from build123d import *

# Parameters (mm, degrees)
F0_R     = 3
F0_R_2   = 1.5
F1_DEPTH = 2
F2_DEPTH = 7
F3_SIZE  = 1


with BuildPart() as f1:
    # F0 (on Top) → F1 (new body)
    with BuildSketch(Plane.XY):
        Circle(F0_R)
        Circle(F0_R_2, mode=Mode.SUBTRACT)
    extrude(amount=F1_DEPTH)

    # F0 (on Top) → F2 (join)
    with BuildSketch(Plane.XY):
        Circle(F0_R_2)
    extrude(amount=F2_DEPTH)

    # F3
    f3_edges = [f1.edges().sort_by_distance(p)[0] for p in [
        (-1.5, 0, 7),
    ]]
    chamfer(f3_edges, length=F3_SIZE)


solid = f1.part
Model file for the job. Use its own axes, mm. A direction names the side the tool comes from. Round coordinates to 2 decimals unless told otherwise and drop trailing zeros. Order: outer loops, then holes, each group sorted by start corner. A loop starts at its lowest first (then second) coordinate and runs counter-clockwise, first axis right, second up. Notation, with made-up numbers: M 53,26 L 70,26 A16 cw 70,46 Z; hole C -20.75,18 d4. An arc over 180 degrees is marked long. Write each question's results on one line, items separated by ' | '. Start each with the question number.
(1) Drop flat-ended pins along their axis: pin 1 (1 mm diameter, centred on y = 1, z = 5, fed in from -X); pin 2 (2 mm diameter, centred on x = -1.5, z = 6, fed in from -Y). Give the stop position or say it passes through.
(2) Which spindle directions (+Z, -Z, +X, -X, +Y, -Y) get a long thin tool onto all of the face, cutting with end or side? Do faces 1 (the face through (1.3, -1.3, 2)), 2 (the face through (-3, 0, 1)). Say none if no direction does.
(3) Probe probe 1 along Z at (x, y) = (0.45, -2.25); probe 2 along Z at (x, y) = (0.7, -0.1); probe 3 along X at (y, z) = (-1.15, 3). List the from-to ranges inside material, lowest first. Write a range as from..to.
(4) Saw through at C-C, the plane z = 6.75. Give the cut face in (x, y), then the cut area to 3 significant figures.
(5) Saw through at A-A, the plane x = 0. Give the cut face in (y, z).
(6) Saw through at D-D, the plane z = 4. Give the cut face in (x, y), then the cut area to 3 significant figures.
Established:
1) pin 1: stops at x = -1.41 | pin 2: stops at y = -1.41
2) face 1: +Z | face 2: +Z, -Z
3) probe 1: z = 0..2 | probe 2: z = 0..6.79 | probe 3: x = -0.96..0.96
4) outline: C 0,0 d1.5 | area: 1.77 mm^2
5) outline: M -3,0 L 3,0 L 3,2 L 1.5,2 L 1.5,6 L 0.5,7 L -0.5,7 L -1.5,6 L -1.5,2 L -3,2 Z
6) outline: C 0,0 d3 | area: 7.07 mm^2
